Autodesk Inventor part; units mm, degrees
ref_plane "YZ Plane" through (0, 0, 0) normal (1, 0, 0) x (0, 1, 0)
ref_plane "XZ Plane" through (0, 0, 0) normal (0, 1, 0) x (-1, 0, 0)
ref_plane "XY Plane" through (0, 0, 0) normal (0, 0, 1) x (1, 0, 0)
sketch "Sketch1" plane through (0, 0, 0) normal (1, 0, 0) x (0, 1, 0)
  circle A0 centre (45, 0) radius 11
  line L0 (45, 0) -> (0, 0)
  circle A1 centre (130, 235) radius 11
  line L1 (73.2002, 0) -> (73.2002, 46.6199)
  line L2 (77.2194, 61.6199) -> (155.9808, 198.0385)
  line L3 (160, 213.0385) -> (160, 235)
  arc A2 (160, 235) -> (130, 265) centre (130, 235) ccw
  line L4 (130, 235) -> (130, 265) construction
  line L5 (130, 235) -> (160, 235) construction
  line L6 (130, 265) -> (-45, 265)
  circle A3 centre (-45, 0) radius 18
  line L7 (0, 0) -> (0, 265)
  circle A4 centre (-45, 235) radius 13
  arc A5 (-45, 265) -> (-75, 235) centre (-45, 235) ccw
  line L8 (-45, 235) -> (-75, 235) construction
  line L9 (-45, 235) -> (-45, 265) construction
  line L10 (-75, 235) -> (-75, 39.1421)
  line L11 (0, 0) -> (-45, 0)
  circle A6 centre (130, -235) radius 11
  line L12 (73.2002, 0) -> (73.2002, -46.6199)
  line L13 (77.2194, -61.6199) -> (155.9808, -198.0385)
  line L14 (160, -213.0385) -> (160, -235)
  arc A7 (130, -265) -> (160, -235) centre (130, -235) ccw
  line L15 (130, -265) -> (-45, -265)
  circle A8 centre (-45, -235) radius 13
  arc A9 (-75, -235) -> (-45, -265) centre (-45, -235) ccw
  line L16 (-45, -235) -> (-75, -235) construction
  line L17 (-75, -235) -> (-75, -39.1421)
  arc A10 (155.9808, 198.0385) -> (160, 213.0385) centre (130, 213.0385) ccw
  arc A11 (77.2194, 61.6199) -> (73.2002, 46.6199) centre (103.2002, 46.6199) ccw
  arc A12 (73.2002, -46.6199) -> (77.2194, -61.6199) centre (103.2002, -46.6199) ccw
  arc A13 (160, -213.0385) -> (155.9808, -198.0385) centre (130, -213.0385) ccw
  line L18 (-77.9289, 32.0711) -> (-82.0711, 27.9289)
  line L19 (-85, 20.8579) -> (-85, 0)
  line L20 (-77.9289, -32.0711) -> (-82.0711, -27.9289)
  line L21 (-85, -20.8579) -> (-85, 0)
  arc A14 (-77.9289, 32.0711) -> (-75, 39.1421) centre (-85, 39.1421) ccw
  arc A15 (-82.0711, 27.9289) -> (-85, 20.8579) centre (-75, 20.8579) ccw
  arc A16 (-85, -20.8579) -> (-82.0711, -27.9289) centre (-75, -20.8579) ccw
  arc A17 (-75, -39.1421) -> (-77.9289, -32.0711) centre (-85, -39.1421) ccw
  point P0 (73.2002, 54.6584)
  point P1 (160, 205)
  point P2 (-75, -35)
  point P3 (48.2002, -10.5242)
  point P4 (73.2002, -54.6584)
  point P5 (160, -205)
  point P6 (-85, 25)
  point P7 (-75, 35)
  point P8 (-85, -25)
  dimension "d0" = 22
  dimension "d1" = 22
  dimension "d2" = 470
  dimension "d3" = 90
  dimension "d4" = 36
  dimension "d7" = 30
  dimension "d8" = 26
  dimension "d9" = 90
  dimension "d11" = 25
  dimension "d12" = 85
  dimension "d13" = 90
  dimension "d14" = 30
  dimension "d15" = 30
  dimension "d16" = 30
  dimension "d19" = 45
  dimension "d20" = 40
  dimension "d21" = 50
  dimension "d22" = 10
extrude "Extrusion1" add sketch "Sketch1" along normal mid plane 25.4
properties part number "Balancim_3-Cabos_Modelo1"
Check sheet for the modelled part. Datum: model origin and axes. Units: mm. A direction names the side the tool comes from. Round coordinates to 2 decimals unless told otherwise and drop trailing zeros. Order: outer loops, then holes, each group sorted by start corner. A loop starts at its lowest first (then second) coordinate and runs counter-clockwise, first axis right, second up. Notation, with made-up numbers: M -14.5,-12.5 L 30.5,-12.5 A28 ccw 30.5,11.5 Z; hole C 6.25,-2 d10. An arc over 180 degrees is marked long. One line per item, written item: value. Start each with the question number.
1. Access from +Z, -Z, +X, -X, +Y, -Y to the whole of each face (thin tool, end or side, straight path). Record for faces 4 (the flat face through (0, -75, -138)), 5 (the flat face through (-0.178, 116.049, -128.874)), 6 (the flat face through (0, -75, 138)).
2. Section check B-B on x = 0.25. Give the number of separate pieces and of enclosed holes in the cut face, and give its area (3 significant figures).
3. Gauge pin test, flat ends, axial feed: P1, Ø20, axis at y = 130, z = -235, coming from the -X side; P2, Ø12.5, axis at x = 5, z = 179, coming from the -Y side; P3, Ø1, axis at x = -1.5, y = -59, coming from the +Z side; P4, Ø8, axis at x = -8.5, y = -55.5, coming from the +Z side. Record the tip position at first contact, or that the pin passes through.
4. Release check for a two-part mould opening along Y. For faces 1 (the cylindrical face through (-0.178, 128.568, -245.906)), 2 (the flat face through (0, 44, 265)), 3 (the cylindrical face through (-0.2, 74.2, 54.3)) record: released by +Y, released by -Y, zero draft, split by the parting line, or undercut.
5. Section check A-A on y = 45. Enter the section's corners in (x, z), and give its area (3 significant figures).
6. Scan lines: line 1 along Z through (x, y) = (-6.25, -45); line 2 along Z through (x, y) = (4, 130); line 3 along Z through (x, y) = (-4.25, 45). Record each from-to range of solid material in increasing order.
7. Section check C-C on z = -86. Enter the section's corners in (x, y).
8. Section check D-D on z = 152.5. Enter the section's corners in (x, y), and give its area (3 significant figures).
Results found:
1. face 4: -Z, +X, -X, -Y
1. face 5: +X, -X, +Y
1. face 6: +Z, +X, -X, -Y
2. separate pieces: 1
2. enclosed holes: 6
2. area: 98,600 mm^2
3. P1: through
3. P2: y = -75
3. P3: z = 261.79
3. P4: z = 264.29
4. face 1: undercut
4. face 2: zero draft
4. face 3: released by +Y
5. outline: M -12.7,-265 L 12.7,-265 L 12.7,-11 L -12.7,-11 Z; M -12.7,11 L 12.7,11 L 12.7,265 L -12.7,265 Z
5. area: 12,900 mm^2
6. line 1: -265 to -248, -222 to -18, 18 to 222, 248 to 265
6. line 2: -265 to -246, -224 to -153.04, 153.04 to 224, 246 to 265
6. line 3: -265 to -11, 11 to 265
7. outline: M -12.7,-75 L 12.7,-75 L 12.7,91.3 L -12.7,91.3 Z
8. outline: M -12.7,-75 L 12.7,-75 L 12.7,129.69 L -12.7,129.69 Z
8. area: 5,200 mm^2
